Could you check a few things on this model? Use its own coordinates, in mm. A direction names the side the tool comes from. Give positions to 0.01 mm unless a question says otherwise; leave off trailing zeros. Loops run counter-clockwise (first coordinate to the right, second up) from the corner with the lowest first, then second, coordinate; pieces in that order, holes last. Notation, with made-up numbers: (60.5, -17.5) - (117.5, -17.5) arc R13 cw to (117.5, 0.5) - close; hole circle Ø6 at (18.5, 86.5). An arc over 180 degrees is marked (long way). Use CSV: the item, a comma, the result in double quotes.
Solid Edge part; units mm, degrees
sketch "Sketch1" plane through (0, 0, 0) normal (0, -1, 0) x (1, 0, 0)
  line L0 (-3, 0) -> (-6, 0)
  line L1 (-6, 0) -> (-6, 2)
  line L2 (-6, 2) -> (-5, 2)
  line L3 (-5, 2) -> (-5, 14)
  line L4 (-5, 14) -> (-4, 26.75)
  line L5 (-4, 26.75) -> (-3.5, 26.75)
  line L6 (-3.5, 26.75) -> (-3.5, 42)
  line L7 (-3.5, 42) -> (0, 42)
  line L8 (0, 23) -> (-3, 23)
  line L9 (-3, 23) -> (-3, 0)
  dimension "D1" = 6
  dimension "D2" = 5
revolve "RevolvedProtrusion1" add sketch "Sketch1" angle 360 about axis through (0, 0, 42) along (0, 0, -1)
fillet "Round1" radius 3.5 1 edges at (3.5, 0, 42)
fillet "Round___Bottom" radius 0.2 1 edges at (5, 0, 2)
chamfer "Chamfer___Inner" distance 1 angle 45 1 edges at (3, 0, 23)
properties material "Stainless Steel, 420"
1) Suppose I cut it at D-D (z = 30.5). Please give me the cut outline in (x, y), plus the area to 3 significant figures.
Answer below:
outline,"circle Ø7 at (0, 0)"
area,"38.5 mm2"
2) Suppose I cut it at C-C (z = 6). Please give me the cut outline in (x, y), plus the area to 3 significant figures.
Answer below:
outline,"circle Ø10 at (0, 0); hole circle Ø6 at (0, 0)"
area,"50.3 mm2"
3) We'd pull the mould along Y, two halves only. Please class faces 4 (the cylindrical face through (6, 0, 1)), 5 (the flat face through (0, 0, 23)), 6 (the flat face through (2, 5, 2)): +Y half, -Y half, draft (parallel to the pull), parting line (faces both ways), or undercut.
Answer below:
face 4,"parting line"
face 5,"undercut"
face 6,"draft"
4) I'm going to push flat-ended pins straight in: P1, Ø4, axis at y = 1.5, z = 29.5, coming from the -X side; P2, Ø4, axis at x = 1.5, y = 1.5, coming from the +Z side; P3, Ø2, axis at x = 0.5, y = 1, coming from the -Z side. Where does each tip first touch, or does it pass through?
Answer below:
P1,"stops at x = -3.5"
P2,"stops at z = 42"
P3,"stops at z = 22.88"
5) I need wall thicknesses on line 1 along Y through (x, z) = (0, 11.25); line 2 along Z through (x, y) = (-4.75, 3.5); line 3 along Y through (x, z) = (0, 16.5). Which ranges of each line are inside material? Lowest first, please.
Answer below:
line 1,"y = -5 to -3, 3 to 5"
line 2,"z = 0 to 2"
line 3,"y = -4.8 to -3, 3 to 4.8"
6) Which directions (+Z, -Z, +X, -X, +Y, -Y) give clear straight access to the entire face, cutting with the end or side of a thin tool? Please do faces 1 (the cylindrical face through (3, 0, 11)), 2 (the cylindrical face through (-3.233, 1.341, 32.707)), 3 (the flat face through (3, -1, 0)).
Answer below:
face 1,"-Z"
face 2,"+Z"
face 3,"-Z, +X, -X, +Y, -Y"
7) Suppose I cut it at A-A (y = 0). Please give me the cut outline in (x, z).
Answer below:
outline,"(-6, 0) - (-3, 0) - (-3, 22) - (-2, 23) - (2, 23) - (3, 22) - (3, 0) - (6, 0) - (6, 2) - (5.2, 2) arc R0.2 cw to (5, 2.2) - (5, 14) - (4, 26.75) - (3.5, 26.75) - (3.5, 38.5) arc R3.5 ccw to (-3.5, 38.5) - (-3.5, 26.75) - (-4, 26.75) - (-5, 14) - (-5, 2.2) arc R0.2 cw to (-5.2, 2) - (-6, 2) - close"
